For this review, take the finished solid that the model builds, in its own axes (mm). A direction names the side the tool comes from. Round coordinates to 2 decimals unless told otherwise and drop trailing zeros. Order: outer loops, then holes, each group sorted by start corner. A loop starts at its lowest first (then second) coordinate and runs counter-clockwise, first axis right, second up. Notation, with made-up numbers: (75.25, 21.5) -> (96.25, 21.5) arc R9 ccw to (96.25, 35.5) -> close; hole circle Ø9 at (-39, -23.5). An arc over 180 degrees is marked (long way). Answer in a Markdown table with one row per item.
```python
from build123d import *

# Parameters (mm, degrees)
SKETCH_1_W           = 8
SKETCH_1_H           = 8
EXTRUDE_1_DEPTH      = 24
FILLET_1_R           = 0.3
HOLE_WIZARD_1_D      = 2.5
HOLE_WIZARD_2_D      = 2.5
HOLE_WIZARD_3_REACH  = 50.332
HOLE_WIZARD_3_BORE_R = 1.25


with BuildPart() as part:
    # 草图1 → 凸台-拉伸1 (new, symmetric)
    with BuildSketch(Plane(origin=(0, 0, 0), x_dir=(0, 0, -1), z_dir=(1, 0, 0))):
        Rectangle(SKETCH_1_W, SKETCH_1_H)
    extrude(amount=EXTRUDE_1_DEPTH, both=True)

    # 圆角1
    fillet_1_edges = [part.edges().sort_by_distance(p)[0] for p in [
        (24, 0, 4),
        (24, -4, 0),
        (24, 0, -4),
        (-24, -4, 0),
        (-24, 0, 4),
        (-24, 4, 0),
        (-24, 0, -4),
        (0, -4, -4),
        (0, -4, 4),
        (0, 4, 4),
        (0, 4, -4),
        (24, 4, 0),
    ]]
    fillet(fillet_1_edges, radius=FILLET_1_R)

    # 螺纹孔1 (through all)
    with Locations(Plane(origin=(0, 4, 0), x_dir=(1, 0, 0), z_dir=(0, 1, 0))):
        with Locations((-8, 0), (8, 0)):
            Hole(HOLE_WIZARD_1_D / 2)

    # 螺纹孔2 (through all)
    with Locations(Plane.XY.offset(4)):
        with Locations((-16, 0), (16, 0)):
            Hole(HOLE_WIZARD_2_D / 2)

    # 螺纹孔3 bore → 螺纹孔3 (cut, up to next)
    with BuildSketch(Plane.ZY.offset(24), mode=Mode.PRIVATE) as hole_wizard_3_sk1:
        Circle(HOLE_WIZARD_3_BORE_R)
    hole_wizard_3_tool1 = extrude(hole_wizard_3_sk1.sketch, amount=-HOLE_WIZARD_3_REACH, mode=Mode.PRIVATE) & part.part
    hole_wizard_3 = hole_wizard_3_tool1.solids().sort_by_distance((-24, 0, 0))[0]
    add(hole_wizard_3, mode=Mode.SUBTRACT)

    # 镜向1: 螺纹孔3 across plane
    add(hole_wizard_3.mirror(Plane(origin=(0, 0, 0), x_dir=(0, 0, 1), z_dir=(1, 0, 0))), mode=Mode.SUBTRACT)


solid = part.part
```
Q1. Take a section at B-B, the plane y = 0. Write out the cut boundary in (x, z), then the cut area to 3 significant figures.
Answer key:
| item | result |
|---|---|
| outline | (-24, -3.7) arc R0.3 ccw to (-23.7, -4) -> (-17.25, -4) -> (-17.25, -1.25) -> (-24, -1.25) -> close; (-24, 1.25) -> (-17.25, 1.25) -> (-17.25, 4) -> (-23.7, 4) arc R0.3 ccw to (-24, 3.7) -> close; (-14.75, -4) -> (14.75, -4) -> (14.75, 4) -> (-14.75, 4) -> close; (17.25, -4) -> (23.7, -4) arc R0.3 ccw to (24, -3.7) -> (24, -1.25) -> (17.25, -1.25) -> close; (17.25, 1.25) -> (24, 1.25) -> (24, 3.7) arc R0.3 ccw to (23.7, 4) -> (17.25, 4) -> close; hole circle Ø2.5 at (-8, 0); hole circle Ø2.5 at (8, 0) |
| area | 300 mm^2 |
Q2. Tool access review of faces 4 (the face through (0, 4, 0)), 5 (the face through (-20.06, 0.05, -1.25)), 6 (the face through (20.06, 0.05, -1.25)): name each direction out of +Z, -Z, +X, -X, +Y, -Y from which nothing blocks a thin tool from reaching the whole face with its end or side.
Answer key:
| item | result |
|---|---|
| face 4 | +Z, -Z, +X, -X, +Y |
| face 5 | -X |
| face 6 | +X |
Q3. Clearance check with flat-ended pins moving along their axes: pin 1 Ø2 at (y, z) = (0, 0) entering from -X; pin 2 Ø1.5 at (x, z) = (8, 0) entering from +Y. State where each tip first meets the part, or that it passes through.
Answer key:
| item | result |
|---|---|
| pin 1 | stops at x = -15.25 |
| pin 2 | passes through |
Q4. To check wall thickness, follow probe 1 along Y at (x, z) = (21, 0); probe 2 along X at (y, z) = (0.75, 3.5). State the ranges of each line that lie inside material, in increasing order.
Answer key:
| item | result |
|---|---|
| probe 1 | y = -4 to -1.25, 1.25 to 4 |
| probe 2 | x = -24 to -17, -15 to 15, 17 to 24 |
Q5. Take a section at C-C, the plane x = 8. Write out the cut boundary in (y, z), then the cut area to 3 significant figures.
Answer key:
| item | result |
|---|---|
| outline | (-4, -3.7) arc R0.3 ccw to (-3.7, -4) -> (3.7, -4) arc R0.3 ccw to (4, -3.7) -> (4, -1.25) -> (-4, -1.25) -> close; (-4, 1.25) -> (4, 1.25) -> (4, 3.7) arc R0.3 ccw to (3.7, 4) -> (-3.7, 4) arc R0.3 ccw to (-4, 3.7) -> close |
| area | 43.9 mm^2 |
Q6. Take a section at D-D, the plane y = -2.75. Write out the cut boundary in (x, z), then the cut area to 3 significant figures.
Answer key:
| item | result |
|---|---|
| outline | (-24, -3.7) arc R0.3 ccw to (-23.7, -4) -> (23.7, -4) arc R0.3 ccw to (24, -3.7) -> (24, 3.7) arc R0.3 ccw to (23.7, 4) -> (-23.7, 4) arc R0.3 ccw to (-24, 3.7) -> close; hole circle Ø2.5 at (-8, 0); hole circle Ø2.5 at (8, 0) |
| area | 374 mm^2 |
Q7. The part is to be moulded in two halves that separate along X. For faces 1 (the face through (24, 0, 2)), 2 (the face through (0, 0, -4)), 3 (the face through (-14.75, 0.05, -0.06)), say which applies: +X half, -X half, draft (parallel to the pull), parting line (faces both ways), or undercut.
Answer key:
| item | result |
|---|---|
| face 1 | +X half |
| face 2 | draft |
| face 3 | undercut |
Q8. Take a section at A-A, the plane z = 0. Write out the cut boundary in (x, y).
Answer key:
| item | result |
|---|---|
| outline | (-24, -3.7) arc R0.3 ccw to (-23.7, -4) -> (-9.25, -4) -> (-9.25, 4) -> (-23.7, 4) arc R0.3 ccw to (-24, 3.7) -> (-24, 1.25) -> (-16, 1.25) arc R1.25 cw to (-16, -1.25) -> (-24, -1.25) -> close; (-6.75, -4) -> (6.75, -4) -> (6.75, 4) -> (-6.75, 4) -> close; (9.25, -4) -> (23.7, -4) arc R0.3 ccw to (24, -3.7) -> (24, -1.25) -> (16, -1.25) arc R1.25 cw to (16, 1.25) -> (24, 1.25) -> (24, 3.7) arc R0.3 ccw to (23.7, 4) -> (9.25, 4) -> close |
